from build123d import *

# Parameters (mm, degrees)
SKETCH_1_W          = 40
SKETCH_1_H          = 39
SKETCH_1_R          = 2
EXTRUDE_1_DEPTH     = 8
SKETCH_2_R          = 1.75
CUT_EXTRUDE_1_DEPTH = 8
CUT_EXTRUDE_START   = -31
SKETCH_2_3_R        = 1.75
CUT_EXTRUDE_2_DEPTH = 8
SKETCH_4_R          = 10
CUT_EXTRUDE_3_DEPTH = 10
CUT_EXTRUDE_5_DEPTH = 10
EXTRUDE_START       = -4
SKETCH_7_R          = 1.6
EXTRUDE_2_DEPTH     = 4


with BuildPart() as part:
    # 草图1 → 凸台-拉伸1 (new body)
    with BuildSketch(Plane(origin=(0, 0, 0), x_dir=(1, 0, 0), z_dir=(0, 1, 0))):
        with Locations((-2, -4)):
            Rectangle(SKETCH_1_W, SKETCH_1_H)
        with Locations(Location((0, 0, 0), (0, 0, 270))):
            Circle(SKETCH_1_R, mode=Mode.SUBTRACT)
    extrude(amount=EXTRUDE_1_DEPTH)

    # 草图2 → 切除-拉伸1 (cut)
    with BuildSketch(Plane.XY.offset(23.5)):
        with Locations((9, 4)):
            Circle(SKETCH_2_R)
        with Locations((-16, 4)):
            Circle(SKETCH_2_R)
    extrude(amount=-CUT_EXTRUDE_1_DEPTH, mode=Mode.SUBTRACT)

    # 草图2<3> → 切除-拉伸2 (cut)
    with BuildSketch(Plane.XY.offset(23.5).offset(CUT_EXTRUDE_START)):
        with Locations((9, 4)):
            Circle(SKETCH_2_3_R)
        with Locations((-16, 4)):
            Circle(SKETCH_2_3_R)
    extrude(amount=-CUT_EXTRUDE_2_DEPTH, mode=Mode.SUBTRACT)

    # 草图4 → 切除-拉伸3 (cut)
    with BuildSketch(Plane(origin=(0, 0, 0), x_dir=(-1, 0, 0), z_dir=(0, -1, 0))):
        with Locations((22, -4)):
            Circle(SKETCH_4_R)
    extrude(amount=-CUT_EXTRUDE_3_DEPTH, mode=Mode.SUBTRACT)

    # 草图6 → 切除-拉伸5 (cut)
    with BuildSketch(Plane(origin=(0, 8, 0), x_dir=(1, 0, 0), z_dir=(0, 1, 0))):
        with BuildLine():
            Line((13, -13.5), (13, 5.5))
            ThreePointArc((13, 5.5), (18, 10.5), (23, 5.5))
            Line((23, 5.5), (23, -13.5))
            ThreePointArc((23, -13.5), (18, -18.5), (13, -13.5))
        make_face()
    extrude(amount=-CUT_EXTRUDE_5_DEPTH, mode=Mode.SUBTRACT)

    # 草图7 → 凸台-拉伸2 (add)
    with BuildSketch(Plane.XZ.offset(EXTRUDE_START)):
        with BuildLine():
            Line((13, -5.5), (13, 13.5))
            ThreePointArc((13, 13.5), (14.464466094, 17.035533906), (18, 18.5))
            Line((18, 18.5), (23, 18.5))
            Line((23, 18.5), (23, -10.5))
            Line((23, -10.5), (18, -10.5))
            ThreePointArc((18, -10.5), (14.464466094, -9.035533906), (13, -5.5))
        make_face()
        with Locations(Location((18, 13.5, 0), (0, 0, 270))):
            Circle(SKETCH_7_R, mode=Mode.SUBTRACT)
        with Locations(Location((18, -5.5, 0), (0, 0, 270))):
            Circle(SKETCH_7_R, mode=Mode.SUBTRACT)
    extrude(amount=EXTRUDE_2_DEPTH)


solid = part.part
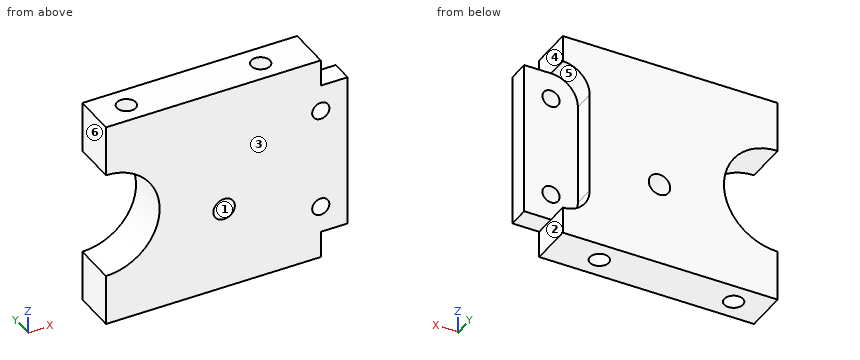
Verification items for the finished model (mm, model axes). Face numbers are marked on the shaded views. A direction names the side the tool comes from. Give positions to 0.01 mm unless a question says otherwise; leave off trailing zeros. Loops run counter-clockwise (first coordinate to the right, second up) from the corner with the lowest first, then second, coordinate; pieces in that order, holes last.
1) Depth check by flat-ended pin: pin 1 Ø5 at (x, z) = (19, -3) entering from +Y; pin 2 Ø2 at (x, y) = (-16, 4) entering from +Z; pin 3 Ø3 at (x, y) = (9, 4) entering from -Z. Enter the tip coordinate at first touch or a pass-through.
2) Thickness scan on line 1 along Y through (x, z) = (-16, 21); line 2 along X through (y, z) = (3, 19.5); line 3 along X through (y, z) = (1.75, 20). Record the ranges inside material, lowest first.
3) Draft check along X on the marked faces 1, 2 and 3. Enter one of: pulls with the +X half, pulls with the -X half, needs draft (parallel to the pull), parting line crosses it, or undercut.
4) Sectioned sample at A-A, the plane x = -16. Enter the section's corners in (y, z).
5) Sectioned sample at C-C, the plane y = 7. Enter the section's corners in (x, z).
6) Sectioned sample at B-B, the plane y = 1.25. Enter the section's corners in (x, z).
7) Set-up check for the marked faces 4, 5 and 6: record each of +Z, -Z, +X, -X, +Y, -Y from which the full face is reachable in a straight line by a thin tool's end or side.
8) Sectioned sample at D-D, the plane z = 0. Enter the section's corners in (x, y), then the cut area to 3 significant figures.
Answers:
1. pin 1: stops at y = 4
1. pin 2: stops at z = 15.5
1. pin 3: stops at z = -7.5
2. line 1: y = 0 to 2.25, 5.75 to 8
2. line 2: x = -22 to -17.44, -14.56 to 7.56, 10.44 to 18
2. line 3: x = -22 to 18
3. face 1: undercut
3. face 2: pulls with the +X half
3. face 3: needs draft
4. outline: (0, -15.5) - (2.25, -15.5) - (2.25, -7.5) - (5.75, -7.5) - (5.75, -15.5) - (8, -15.5) - (8, -4) - (0, -4) - close; (0, 12) - (8, 12) - (8, 23.5) - (5.75, 23.5) - (5.75, 15.5) - (2.25, 15.5) - (2.25, 23.5) - (0, 23.5) - close
5. outline: (-22, -15.5) - (18, -15.5) - (18, -10.5) arc R5 cw to (13, -5.5) - (13, 13.5) arc R5 cw to (18, 18.5) - (18, 23.5) - (-22, 23.5) - (-22, 14) arc R10 cw to (-22, -6) - close; hole circle Ø4 at (0, 0)
6. outline: (-22, -15.5) - (18, -15.5) - (18, -10.5) - (23, -10.5) - (23, 18.5) - (18, 18.5) - (18, 23.5) - (-22, 23.5) - (-22, 14) arc R10 cw to (-22, -6) - close; hole circle Ø4 at (0, 0); hole circle Ø3.2 at (18, -5.5); hole circle Ø3.2 at (18, 13.5)
7. face 4: +Z, +X, +Y, -Y
7. face 5: +X, +Y
7. face 6: +Z, -Z, -X, +Y, -Y
8. outline: (-12.83, 0) - (-2, 0) - (-2, 8) - (-12.83, 8) - close; (2, 0) - (23, 0) - (23, 4) - (13, 4) - (13, 8) - (2, 8) - close
8. area: 215 mm2
